Source: CAD feature listing. Evaluate the final solid. Frame: model axes, mm. A direction names the side the tool comes from. Coordinates: 2 decimals unless noted, no trailing zeros. Write each loop counter-clockwise with the first axis right and the second up, starting at its lowest first coordinate (ties: lowest second). Pieces come first, ordered by that corner, then holes. Notation, with made-up numbers: (69, 75) -> (77, 75) arc R21 cw to (77, 97) -> close; hole circle Ø10 at (2, 14.25). An arc over 180 degrees is marked (long way). Write item = value, one per line.
from build123d import *

# Parameters (mm, degrees)
F0_R     = 9
F1_DEPTH = 140
F2_DEPTH = 70
F3_SIZE  = 31
F4_SIZE  = 0.99999
F5_COUNT = 5
F0_R_2   = 2.25
F6_DEPTH = 62.5
F7_START = 63
F0_R_3   = 7.5
F7_DEPTH = 2


# Not quite as in the source:
# - a fillet or chamfer is up to 0.001 mm smaller than in the source, because OpenCascade refuses the exact size


with BuildPart() as f1:
    # F0 (on Top) → F1 (new body)
    with BuildSketch(Plane.XY):
        with BuildLine():
            ThreePointArc((3, -9.5393920142), (8.0622577483, -5.9160797831), (10, 0))
            ThreePointArc((10, 0), (7.4161984871, 6.7082039325), (1, 9.9498743711))
            ThreePointArc((1, 9.9498743711), (0, 10), (-1, 9.9498743711))
            ThreePointArc((-1, 9.9498743711), (-9.9477573381, 1.0208447195), (-3, -9.5393920142))
            ThreePointArc((-3, -9.5393920142), (-1.5175770051, -9.8841772563), (-2.49e-08, -10))
            ThreePointArc((-2.49e-08, -10), (1.5175769805, -9.8841772601), (3, -9.5393920142))
        make_face()
        Circle(F0_R, mode=Mode.SUBTRACT)
    extrude(amount=F1_DEPTH)

    # F0 (on Top) → F2 (join)
    with BuildSketch(Plane.XY):
        with BuildLine():
            ThreePointArc((-1, 9.9498743711), (0, 10), (1, 9.9498743711))
            Line((1, 9.9498743711), (1, 42.4498743711))
            Line((1, 42.4498743711), (-1, 42.4498743711))
            Line((-1, 42.4498743711), (-1, 9.9498743711))
        make_face()
    extrude(amount=F2_DEPTH)

    # F3
    f3_edges = [f1.edges().sort_by_distance(p)[0] for p in [
        (0, 42.449874, 70),
    ]]
    chamfer(f3_edges, length=F3_SIZE)

    # F4 (size 1 in the source; OpenCascade refuses exactly that, so slightly less here)
    f4_edges = [f1.edges().sort_by_distance(p)[0] for p in [
        (-1, 26.949874, 54.5),
        (1, 26.949874, 54.5),
    ]]
    chamfer(f4_edges, length=F4_SIZE)

    # F5: F1 ×5 about axis
    f5_axis = Axis((0, 0, 0), (0, 0, -1))


with BuildPart() as f1_1:
    add(f1.part)
    for i in range(1, F5_COUNT):
        add(f1.part.rotate(f5_axis, i * 360 / F5_COUNT))

    # F0 (on Top) → F6 (join)
    with BuildSketch(Plane.XY):
        with BuildLine():
            ThreePointArc((-3, -13), (-2.1213203524, -10.8786796652), (-2.49e-08, -10))
            ThreePointArc((-2.49e-08, -10), (-1.5175770051, -9.8841772563), (-3, -9.5393920142))
            Line((-3, -9.5393920142), (-3, -13))
        make_face()
        with BuildLine():
            Line((3, -13), (3, -9.5393920142))
            ThreePointArc((3, -9.5393920142), (1.5175769805, -9.8841772601), (-2.49e-08, -10))
            ThreePointArc((-2.49e-08, -10), (2.1213203348, -10.8786796476), (3, -13))
        make_face()
        with BuildLine():
            ThreePointArc((3, -13), (2.1213203348, -10.8786796476), (-2.49e-08, -10))
            ThreePointArc((-2.49e-08, -10), (-2.1213203524, -10.8786796652), (-3, -13))
            ThreePointArc((-3, -13), (0, -16), (3, -13))
        make_face()
        with Locations((0, -13)):
            Circle(F0_R_2, mode=Mode.SUBTRACT)
    extrude(amount=F6_DEPTH)

    # F0 (on Top) → F7 (join)
    with BuildSketch(Plane.XY.offset(F7_START)):
        Circle(F0_R)
        Circle(F0_R_3, mode=Mode.SUBTRACT)
    extrude(amount=F7_DEPTH)


solid = f1_1.part
1) First-contact query: pin 1 Ø1 at (x, y) = (-1, 23.5) entering from +Z; pin 2 Ø8 at (x, z) = (-2.5, 57) entering from +Y; pin 3 Ø10 at (y, z) = (-0.5, 91.5) entering from -X; pin 4 Ø11 at (x, y) = (0, 0) entering from +Z. Flat tips, straight axial feed; report the tip coordinate or a pass-through.
Answer block:
pin_1 = 57.4
pin_2 = 27.57
pin_3 = -10
pin_4 = through
2) Material intervals for probe 1 along Y at (x, z) = (0, 30); probe 2 along Y at (x, z) = (0, 91); probe 3 along X at (y, z) = (-4, 87), sorted ascending. Write a range as [from, to].
Answer block:
probe_1 = [-16, -15.25], [-10.75, -9], [9, 42.45]
probe_2 = [-10, -9], [9, 10]
probe_3 = [-9.17, -8.06], [8.06, 9.17]
3) Pull-direction query (Y, two-part tool) for faces 4 (the flat face through (-2, 7.4, 65)), 5 (the flat face through (-14.725, -21.968, 26.732)), 6 (the flat face through (25.35, 8.77, 53.91)); classes: +Y half, -Y half, draft (parallel to the pull), parting line (faces both ways), or undercut.
Answer block:
face_4 = undercut
face_5 = -Y half
face_6 = +Y half
4) Cut plane A-A, the plane z = 76. Output: boundary loops of the cut face in (x, y), and give its area (3 significant figures).
Answer block:
outline = circle Ø20 at (0, 0); hole circle Ø18 at (0, 0)
area = 59.7 mm2
5) Reachability of faces 1 (the flat face through (16.34, -20.79, 26.73)), 2 (the cylindrical face through (-1.172, 8.923, 31.059)), 3 (the flat face through (-15.353, -21.994, 53.915)) from +Z, -Z, +X, -X, +Y, -Y: full face, straight path, thin tool, end or side. Return the list, or none.
Answer block:
face_1 = +Z, -Z, +X
face_2 = -Z
face_3 = +Z, -Y
